Part model, mm, in its own coordinate system. A direction names the side the tool comes from. Round coordinates to 2 decimals unless told otherwise and drop trailing zeros. Order: outer loops, then holes, each group sorted by start corner. A loop starts at its lowest first (then second) coordinate and runs counter-clockwise, first axis right, second up. Notation, with made-up numbers: (-30, 48) - (21, 48) arc R26 cw to (21, 83) - close; hole circle Ø10 at (79, 28.5). An arc over 180 degrees is marked (long way). Return JSON: item names as keys, results as strings. Group by question number.
Item 1: Drop flat-ended pins along their axis: pin 1 (5 mm diameter, centred on x = 65, z = -18, fed in from -Y); pin 2 (4 mm diameter, centred on y = 34.5, z = -3, fed in from +X); pin 3 (5.5 mm diameter, centred on x = 49, z = -18.5, fed in from +Y). Give the stop position or say it passes through.
Item 2: Tool access for faces 4 (the face through (19, -3, -20)), 5 (the face through (8, 36, -25)), 6 (the face through (24, -3, -20)), 7 (the face through (63, 5, -17)), 8 (the face through (40, 35, -4)): list every direction of +Z, -Z, +X, -X, +Y, -Y with a clear straight run to the whole face (end or side of a thin tool).
Item 3: Two-plate mould, pull along X, no slides. Class faces 1 (the face through (53.47, 7.54, -18.46)), 2 (the face through (77.15, 5.07, -3.01)), 3 (the face through (14, 0, -20)): released by +X, released by -X, zero draft, split by the parting line, or undercut.
Item 4: Saw through at B-B on y = 27. List the corners of the cut face in (x, z), and give its area (3 significant figures).
Item 5: Saw through at C-C on x = 14. List the corners of the cut face in (y, z), and give its area (3 significant figures).
Item 6: Saw through at D-D on y = 2.5. List the corners of the cut face in (x, z).
Item 7: Probe probe 1 along Z at (x, y) = (50, 2); probe 2 along X at (y, z) = (1.15, -18); probe 3 along X at (y, z) = (42.5, -3). List the from-to ranges inside material, lowest first.
Item 8: Saw through at A-A on x = 65. List the corners of the cut face in (y, z), and give its area (3 significant figures).
```python
from build123d import *

# Parameters (mm, degrees)
SKETCH1_W           = 80
SKETCH1_H           = 40
SKETCH1_R           = 1.6
BOSS_EXTRUDE1_DEPTH = 10
SKETCH2_W           = 8
SKETCH2_H           = 32
SKETCH2_H_2         = 8
SKETCH2_W_2         = 32
BOSS_EXTRUDE2_DEPTH = 50
FILLET1_R           = 10
FILLET2_R           = 3
SKETCH3_R           = 3.5
CUT_EXTRUDE1_DEPTH  = 5
FILLET3_R           = 10
SKETCH4_W           = 5
SKETCH4_H           = 40
BOSS_EXTRUDE3_DEPTH = 5
FILLET4_R           = 1
SKETCH5_R           = 1.5
CUT_EXTRUDE2_DEPTH  = 80


with BuildPart() as part:
    # Sketch1 → Boss-Extrude1 (new body)
    with BuildSketch(Plane(origin=(0, 0, 0), x_dir=(1, 0, 0), z_dir=(0, 1, 0))):
        with Locations((40, 20)):
            Rectangle(SKETCH1_W, SKETCH1_H)
        with Locations(Location((65, 30, 0), (0, 0, 270))):
            Circle(SKETCH1_R, mode=Mode.SUBTRACT)
        with Locations(Location((50, 30, 0), (0, 0, 270))):
            Circle(SKETCH1_R, mode=Mode.SUBTRACT)
        with Locations(Location((50, 18, 0), (0, 0, 270))):
            Circle(SKETCH1_R, mode=Mode.SUBTRACT)
        with Locations(Location((65, 18, 0), (0, 0, 270))):
            Circle(SKETCH1_R, mode=Mode.SUBTRACT)
    extrude(amount=BOSS_EXTRUDE1_DEPTH)

    # Sketch2 → Boss-Extrude2 (add)
    with BuildSketch(Plane(origin=(0, 10, 0), x_dir=(1, 0, 0), z_dir=(0, 1, 0))):
        with Locations((4, 24)):
            Rectangle(SKETCH2_W, SKETCH2_H)
        with Locations((4, 4)):
            Rectangle(SKETCH2_W, SKETCH2_H_2)
        with Locations((24, 4)):
            Rectangle(SKETCH2_W_2, SKETCH2_H_2)
    extrude(amount=BOSS_EXTRUDE2_DEPTH)

    # Fillet1
    fillet1_edges = [part.edges().sort_by_distance(p)[0] for p in [
        (40, 10, -4),
        (40, 60, -4),
        (4, 60, -40),
        (80, 5, -40),
        (80, 5, 0),
    ]]
    fillet(fillet1_edges, radius=FILLET1_R)

    # Fillet2
    fillet2_edges = [part.edges().sort_by_distance(p)[0] for p in [
        (8, 10, -24),
        (8, 35, -8),
        (29, 10, -8),
    ]]
    fillet(fillet2_edges, radius=FILLET2_R)

    # Sketch3 → Cut-Extrude1 (cut)
    with BuildSketch(Plane(origin=(0, 10, 0), x_dir=(1, 0, 0), z_dir=(0, 1, 0))):
        with Locations(Location((50, 30, 0), (0, 0, 270))):
            Circle(SKETCH3_R)
        with Locations(Location((50, 18, 0), (0, 0, 270))):
            Circle(SKETCH3_R)
        with Locations(Location((65, 18, 0), (0, 0, 270))):
            Circle(SKETCH3_R)
        with Locations(Location((65, 30, 0), (0, 0, 270))):
            Circle(SKETCH3_R)
    extrude(amount=-CUT_EXTRUDE1_DEPTH, mode=Mode.SUBTRACT)

    # Fillet3
    fillet3_edges = [part.edges().sort_by_distance(p)[0] for p in [
        (0, 0, -20),
    ]]
    fillet(fillet3_edges, radius=FILLET3_R)

    # Sketch4 → Boss-Extrude3 (add)
    with BuildSketch(Plane.XZ):
        with Locations((21.5, -20)):
            Rectangle(SKETCH4_W, SKETCH4_H)
    extrude(amount=BOSS_EXTRUDE3_DEPTH)

    # Fillet4
    fillet4_edges = [part.edges().sort_by_distance(p)[0] for p in [
        (19, 0, -20),
        (24, 0, -20),
    ]]
    fillet(fillet4_edges, radius=FILLET4_R)

    # Sketch5 → Cut-Extrude2 (cut)
    with BuildSketch(Plane.ZY):
        with Locations((-30, 50)):
            Circle(SKETCH5_R)
        with Locations((-20, 50)):
            Circle(SKETCH5_R)
    extrude(amount=-CUT_EXTRUDE2_DEPTH, mode=Mode.SUBTRACT)


solid = part.part
```
Filled in:
{
 "1": {"pin 1": "stops at y = 0", "pin 2": "stops at x = 40", "pin 3": "stops at y = 10"},
 "2": {"face 4": "+Z, -Z, -X, -Y", "face 5": "-Z, +X, +Y", "face 6": "+Z, -Z, +X, -Y", "face 7": "+Y", "face 8": "+Z, -Z, +X, +Y"},
 "3": {"face 1": "undercut", "face 2": "released by +X", "face 3": "zero draft"},
 "4": {"outline": "(0, -40) - (8, -40) - (8, -11) arc R3 cw to (11, -8) - (40, -8) - (40, 0) - (0, 0) - close", "area": "578 mm^2"},
 "5": {"outline": "(0, -40) - (10, -40) - (10, -11) arc R3 cw to (13, -8) - (60, -8) - (60, 0) - (0, 0) - close", "area": "802 mm^2"},
 "6": {"outline": "(3.39, -40) - (70, -40) arc R10 ccw to (80, -30) - (80, -10) arc R10 ccw to (70, 0) - (3.39, 0) - close; hole circle Ø3.2 at (50, -30); hole circle Ø3.2 at (50, -18); hole circle Ø3.2 at (65, -30); hole circle Ø3.2 at (65, -18)"},
 "7": {"probe 1": "z = -40 to -31.6, -28.4 to -19.6, -16.4 to 0", "probe 2": "x = 5.34 to 48.4, 51.6 to 63.4, 66.6 to 80", "probe 3": "x = 0 to 40"},
 "8": {"outline": "(0, -40) - (10, -40) - (10, -33.5) - (5, -33.5) - (5, -31.6) - (0, -31.6) - close; (0, -28.4) - (5, -28.4) - (5, -26.5) - (10, -26.5) - (10, -21.5) - (5, -21.5) - (5, -19.6) - (0, -19.6) - close; (0, -16.4) - (5, -16.4) - (5, -14.5) - (10, -14.5) - (10, 0) - (0, 0) - close", "area": "298 mm^2"}
}
